For this review, take the finished solid that the model builds, in its own axes (mm). A direction names the side the tool comes from. Coordinates: 2 decimals unless noted, no trailing zeros. Write each loop counter-clockwise with the first axis right and the second up, starting at its lowest first coordinate (ties: lowest second). Pieces come first, ordered by that corner, then holes.
```python
from build123d import *

# Parameters (mm, degrees)
SKETCH_2_R               = 5.5
EXTRUDE_671_DEPTH        = 12
SKETCH_3_R               = 5.5
EXTRUDE_1_DEPTH          = 15
SKETCH_4_R               = 31
EXTRUDE_2_DEPTH          = 22
EXTRUDE_2_TAPER          = 3
CUT_EXTRUDE_2_DEPTH      = 3
PATTERN_CIRCULAR_1_COUNT = 2
SKETCH_11_W              = 31
SKETCH_11_H              = 3.915
SKETCH_12_W              = 0.2
SKETCH_12_H              = 4.725
SKETCH_13_W              = 2.567
SKETCH_13_H              = 15.915


with BuildPart() as part:
    # 草图2 → Extrude 671 (new body)
    with BuildSketch(Plane.XY):
        with BuildLine():
            Line((-49.983333333, 10.364187807), (-13.433333333, 27.938245391))
            ThreePointArc((-13.433333333, 27.938245391), (0, 31), (13.433333333, 27.938245391))
            Line((13.433333333, 27.938245391), (49.983333333, 10.364187807))
            ThreePointArc((49.983333333, 10.364187807), (56.5, 0), (49.983333333, -10.364187807))
            Line((49.983333333, -10.364187807), (13.433333333, -27.938245391))
            ThreePointArc((13.433333333, -27.938245391), (0, -31), (-13.433333333, -27.938245391))
            Line((-13.433333333, -27.938245391), (-49.983333333, -10.364187807))
            ThreePointArc((-49.983333333, -10.364187807), (-56.5, 0), (-49.983333333, 10.364187807))
        make_face()
        with Locations((-45, 0)):
            Circle(SKETCH_2_R, mode=Mode.SUBTRACT)
        with Locations(Location((45, 0, 0), (0, 0, 180))):
            Circle(SKETCH_2_R, mode=Mode.SUBTRACT)
    extrude(amount=EXTRUDE_671_DEPTH)

    # 草图3 → 凸台-拉伸1 (add)
    with BuildSketch(Plane.XY):
        with BuildLine():
            Line((-45, 11.5), (45, 11.5))
            ThreePointArc((45, 11.5), (56.5, 0), (45, -11.5))
            Line((45, -11.5), (-45, -11.5))
            ThreePointArc((-45, -11.5), (-56.5, 0), (-45, 11.5))
        make_face()
        with Locations(Location((45, 0, 0), (0, 0, 180))):
            Circle(SKETCH_3_R, mode=Mode.SUBTRACT)
        with Locations((-45, 0)):
            Circle(SKETCH_3_R, mode=Mode.SUBTRACT)
    extrude(amount=EXTRUDE_1_DEPTH)

    # 草图4 → 凸台-拉伸2 (add)
    with BuildSketch(Plane.XY.offset(12)):
        Circle(SKETCH_4_R)
    extrude(amount=EXTRUDE_2_DEPTH, taper=EXTRUDE_2_TAPER)

    # 草图5 → 切除-拉伸2 (cut)
    with BuildSketch(Plane(origin=(0, 0, 0), x_dir=(-1, 0, 0), z_dir=(0, 0, -1))):
        with BuildLine():
            Line((-34.96012629, 11.740142073), (-11.149666667, 23.188743675))
            ThreePointArc((-11.149666667, 23.188743675), (0, 25.73), (11.149666667, 23.188743675))
            Line((11.149666667, 23.188743675), (34.96012629, 11.740142073))
            ThreePointArc((34.96012629, 11.740142073), (36.584583298, 9.705433588), (36.006307058, 7.166832443))
            ThreePointArc((36.006307058, 7.166832443), (33.5, 0), (36.006307058, -7.166832443))
            ThreePointArc((36.006307058, -7.166832443), (36.584583298, -9.705433588), (34.96012629, -11.740142073))
            Line((34.96012629, -11.740142073), (11.149666667, -23.188743675))
            ThreePointArc((11.149666667, -23.188743675), (0, -25.73), (-11.149666667, -23.188743675))
            Line((-11.149666667, -23.188743675), (-34.96012629, -11.740142073))
            ThreePointArc((-34.96012629, -11.740142073), (-36.584583298, -9.705433588), (-36.006307058, -7.166832443))
            ThreePointArc((-36.006307058, -7.166832443), (-33.5, 0), (-36.006307058, 7.166832443))
            ThreePointArc((-36.006307058, 7.166832443), (-36.584583298, 9.705433588), (-34.96012629, 11.740142073))
        make_face()
    extrude(amount=-CUT_EXTRUDE_2_DEPTH, mode=Mode.SUBTRACT)

    # 草图6 → 切除-旋转1 (revolve, cut)
    with BuildSketch(Plane(origin=(0, 0, 0), x_dir=(0, 0, -1), z_dir=(1, 0, 0))):
        with BuildLine():
            Line((-36, 26), (-28.5, 26))
            ThreePointArc((-28.5, 26), (-26.732233047, 25.267766953), (-26, 23.5))
            Line((-26, 23.5), (-26, 22.433234274))
            ThreePointArc((-26, 22.433234274), (-24.841010415, 22.762526163), (-23.666666667, 23.031982594))
            Line((-23.666666667, 23.031982594), (-23.666666667, 25.267766953))
            Line((-23.666666667, 25.267766953), (-21.333333333, 25.267766953))
            Line((-21.333333333, 25.267766953), (-21.333333333, 23.383873836))
            ThreePointArc((-21.333333333, 23.383873836), (-16.618745428, 23.379042467), (-12, 22.433234274))
            Line((-12, 22.433234274), (-12, 23.5))
            ThreePointArc((-12, 23.5), (-11.267766953, 25.267766953), (-9.5, 26))
            Line((-9.5, 26), (2, 26))
            Line((2, 26), (2, 0))
            Line((2, 0), (-36, 0))
            Line((-36, 0), (-36, 26))
        make_face()
    revolve(axis=Axis((0, 0, 0), (0, 0, 1)), mode=Mode.SUBTRACT)

    # 草图7 → 凸台-旋转1 (revolve)
    with BuildSketch(Plane.XY.offset(18.5)):
        with BuildLine():
            Line((-21.679433892, -21.679433892), (-18.850924901, -24.507942884))
            Line((-18.850924901, -24.507942884), (-19.156642158, -24.813660141))
            ThreePointArc((-19.156642158, -24.813660141), (-19.904442449, -25.676726722), (-20.521738978, -26.637473407))
            ThreePointArc((-20.521738978, -26.637473407), (-22.766611284, -28.272961601), (-25.455384104, -27.576704447))
            Line((-25.455384104, -27.576704447), (-26.0493538, -26.982734751))
            ThreePointArc((-26.0493538, -26.982734751), (-26.516044275, -27.176044275), (-26.982734751, -26.982734751))
            Line((-26.982734751, -26.982734751), (-21.679433892, -21.679433892))
        make_face()
    revolve(axis=Axis((-26.982734751, -26.982734751, 18.5), (0.7071067811865517, 0.7071067811865434, 0)))

    # 草图8 → 凸台-旋转2 (revolve)
    with BuildSketch(Plane(origin=(0, 0, 0), x_dir=(0, 0, -1), z_dir=(1, 0, 0)), mode=Mode.PRIVATE) as revolve_2_sk:
        with BuildLine():
            Line((-26, 22.433234274), (-26, 18.64))
            Line((-26, 18.64), (-12, 18.64))
            Line((-12, 18.64), (-12, 22.433234274))
            ThreePointArc((-12, 22.433234274), (-19, 23.5), (-26, 22.433234274))
        make_face()
    revolve(revolve_2_sk.sketch.rotate(Axis((0, 0, 19), (0, 0, -1)), 180), axis=Axis((0, 0, 19), (0, 0, -1)))

    # 草图9 → 凸台-旋转3 (revolve)
    with BuildSketch(Plane(origin=(0, 0, 0), x_dir=(0, 0, -1), z_dir=(1, 0, 0))):
        with BuildLine():
            Line((-19, 20.5975), (-19, 12.9025))
            ThreePointArc((-19, 12.9025), (-15.1525, 16.75), (-19, 20.5975))
        make_face()
    revolve_3 = revolve(axis=Axis((0, 0, 19), (0, 1, 0)))

    # 阵列(圆周)1: 凸台-旋转3 ×2 about axis
    pattern_circular_1_axis = Axis((0, 0, 0), (0, 0, 1))
    for i in range(1, PATTERN_CIRCULAR_1_COUNT):
        add(revolve_3.rotate(pattern_circular_1_axis, i * 360 / PATTERN_CIRCULAR_1_COUNT))

    # 草图11 → 凸台-旋转4 (revolve)
    with BuildSketch(Plane(origin=(0, 0, 0), x_dir=(0, 0, -1), z_dir=(1, 0, 0)), mode=Mode.PRIVATE) as revolve_4_sk:
        with Locations((-21.8, 11.9575)):
            Rectangle(SKETCH_11_W, SKETCH_11_H)
    revolve(revolve_4_sk.sketch.rotate(Axis((0, 0, 19), (0, 0, -1)), 180), axis=Axis((0, 0, 19), (0, 0, -1)))

    # 草图12 → 凸台-旋转5 (revolve)
    with BuildSketch(Plane(origin=(0, 0, 0), x_dir=(0, 0, -1), z_dir=(1, 0, 0)), mode=Mode.PRIVATE) as revolve_5_sk:
        with Locations((-25.7, 16.4775)):
            Rectangle(SKETCH_12_W, SKETCH_12_H)
        with Locations((-12.3, 16.4775)):
            Rectangle(SKETCH_12_W, SKETCH_12_H)
    revolve(revolve_5_sk.sketch.rotate(Axis((0, 0, 0), (0, 0, 1)), 180), axis=Axis((0, 0, 0), (0, 0, 1)))

    # 草图13 → 切除-旋转2 (revolve, cut)
    with BuildSketch(Plane(origin=(0, 0, 0), x_dir=(0, 0, -1), z_dir=(1, 0, 0)), mode=Mode.PRIVATE) as cut_revolve_2_sk:
        with Locations((-31.0165, 7.9575)):
            Rectangle(SKETCH_13_W, SKETCH_13_H)
    revolve(cut_revolve_2_sk.sketch.rotate(Axis((0, 15.915, 32.3), (0, -1, 0)), 180), axis=Axis((0, 15.915, 32.3), (0, -1, 0)), mode=Mode.SUBTRACT)


solid = part.part
```
1) Tool access review of faces 1 (the face through (-18, 7, 26)), 2 (the face through (24.6, -16.72, 1.48)), 3 (the face through (14, -3, 12.4)): name each direction out of +Z, -Z, +X, -X, +Y, -Y from which nothing blocks a thin tool from reaching the whole face with its end or side.
2) Consider section A-A (z = 32.3). Give the boundary of the cut face in (x, y) (3 decimals), then the cut area to 3 significant figures.
3) The part is to be moulded in two halves that separate along X. For faces 4 (the face through (-31.96, 19.03, 5.92)), 5 (the face through (0, 31, 6)), 6 (the face through (36.576, -9.742, 1.479)), say which applies: pulls with the +X half, pulls with the -X half, needs draft (parallel to the pull), parting line crosses it, or undercut.
4) Consider section D-D (x = 47.5). Give the boundary of the cut face in (y, z).
5) For L1, parallel to X at y = -9, z = 10.5; L2, parallel to X at y = -12.5, z = 13; L3, parallel to Y at x = 10.5, z = 19.5, list the stretches that pass through material, from the lowest coordinate up.
6) Consider section B-B (x = 0). Count the separate pieces of the cut face and the enclosed holes in it, then the cut area to 3 significant figures.
7) Clearance check with flat-ended pins moving along their axes: P1, Ø3.5, axis at x = 38, z = 13.5, coming from the -Y side; P2, Ø2, axis at y = 19, z = 12, coming from the +X side; P3, Ø3.5, axis at x = 40, z = 13, coming from the +Y side; P4, Ø9, axis at x = -35.5, y = -23, coming from the +Z side. State where each tip first meets the part, or that it passes through.
Results:
1. face 1: +Z
1. face 2: -Z
1. face 3: none
2. outline: circle Ø59.872 at (0, 0); (-2.567, 9.665) - (-2.567, 13.676) arc R13.915 ccw (long way) to (2.567, 13.676) - (2.567, 9.665) arc R10 cw (long way) to start; hole circle Ø52 at (0, 0)
2. area: 966 mm2
3. face 4: pulls with the -X half
3. face 5: parting line crosses it
3. face 6: undercut
4. outline: (-11.56, 0) - (-4.9, 0) - (-4.9, 15) - (-11.22, 15) - (-11.22, 12) - (-11.56, 12) - close; (4.9, 0) - (11.56, 0) - (11.56, 12) - (11.22, 12) - (11.22, 15) - (4.9, 15) - close
5. L1: x = -52.16 to -24.17, -10.61 to -4.36, 4.36 to 10.61, 24.17 to 52.16
5. L2: x = -28.31 to -13.83, -6.11 to 6.11, 13.83 to 28.31
5. L3: y = -28.75 to -15.4, -9.13 to 9.13, 15.4 to 28.75
6. separate pieces: 3
6. enclosed holes: 2
6. area: 810 mm2
7. P1: stops at y = -16.56
7. P2: stops at x = 34.1
7. P3: stops at y = 15.85
7. P4: passes through
